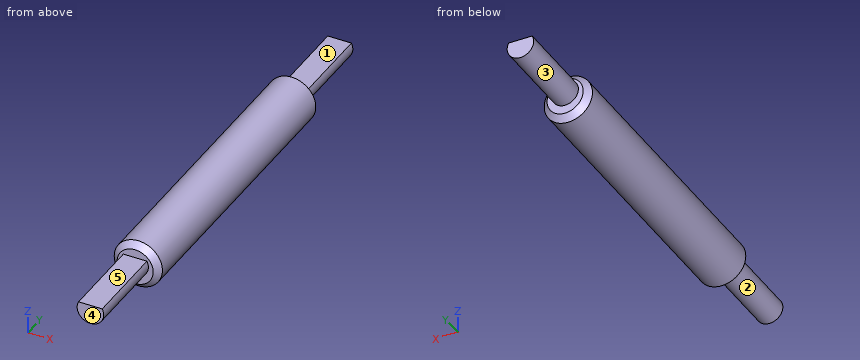
Autodesk Inventor part; units mm, degrees
ref_plane "XZ Plane" through (0, 0, 0) normal (0, 1, 0) x (-1, 0, 0)
ref_plane "XY Plane" through (0, 0, 0) normal (0, 0, 1) x (1, 0, 0)
sketch "Sketch1" plane through (0, 0, 0) normal (0, 1, 0) x (-1, 0, 0)
  circle A0 centre (0, 0) radius 2
  dimension "d0" = 4
extrude "Extrusion1" add sketch "Sketch1" along normal blind 25
sketch "Sketch2" plane through (0, 25, 0) normal (0, 1, 0) x (1, 0, 0)
  line L0 (0, -2) -> (2.3553, -2)
  line L1 (-0.9798, -0.8) -> (0.9798, -0.8)
  arc A0 (0.9798, -0.8) -> (-0.9798, -0.8) centre (0, -0.3) ccw
  circle A1 centre (0, 0) radius 2
  line L2 (3.2263, 0) -> (-2.8711, 0)
  dimension "d4" = 1.2
  dimension "d6" = 1.1
  dimension "d7" = 0.3
extrude "Extrusion2" add sketch "Sketch2" along normal blind 7 contours A0 L2 L1 | A0 L2
sketch "Sketch3" plane through (0, 0, 0) normal (0, -1, 0) x (1, 0, 0)
  line L0 (-0.9798, 0.8) -> (0.9798, 0.8)
  arc A0 (-0.9798, 0.8) -> (0.9798, 0.8) centre (0, 0.3) ccw
  point P0 (0, 0)
  point P1 (0, 0)
  point P2 (0, 0.8)
  dimension "d12" = 1.9596
  dimension "d16" = 1.1
  dimension "d17" = 0.3
extrude "Extrusion3" add sketch "Sketch3" along normal blind 7
chamfer "Chamfer1" distance 0.5 angle 45 1 edges at (2, 25, 0)
chamfer "Chamfer2" distance 0.5 angle 45 1 edges at (2, 0, 0)
equation "\"d4\" = d3"
properties part number "axle-skibidi"
Check sheet for the modelled part. Datum: model origin and axes. Units: mm. Face numbers are marked on the shaded views. A direction names the side the tool comes from. Coordinates: 2 decimals unless noted, no trailing zeros. Loops run counter-clockwise (first coordinate to the right, second up) from the corner with the lowest first, then second, coordinate; pieces in that order, holes last. Notation, with made-up numbers: (-23.5, -27) -> (11.5, -27) arc R21 ccw to (11.5, -5) -> close; hole circle Ø5 at (89, -5.75). An arc over 180 degrees is marked (long way). Write item = value, one per line. Start each with the question number.
1. Tool access check on the marked faces 1, 2, 3, 4 and 5. Record the directions out of +Z, -Z, +X, -X, +Y, -Y that give a thin tool (end or side, any length) a straight path to the whole face; none if there is none.
2. Material ranges on line 1 (Y direction, x = -1.4, z = 0.5); line 2 (Z direction, x = -0.5, y = 18.5); line 3 (Z direction, x = -0.9, y = 1.5), recorded low to high.
3. Section check D-D on y = 22.5. Record the cut outline in (x, z), then the cut area to 3 significant figures.
4. Depth check by flat-ended pin: P1, Ø2, axis at x = -0.5, y = 27, coming from the +Z side. Enter the tip coordinate at first touch or a pass-through.
5. Section check A-A on x = 0. Record the cut outline in (y, z).
6. Section check C-C on y = -2. Record the cut outline in (x, z), then the cut area to 3 significant figures.
7. Section check B-B on z = 0. Record the cut outline in (x, y), then the cut area to 3 significant figures.
Responses:
q1.face_1 = +Z, +X, -X, +Y
q1.face_2 = -Y
q1.face_3 = +Y
q1.face_4 = +Z, -Z, +X, -X, -Y
q1.face_5 = +Z, +X, -X, -Y
q2.line_1 = 0 to 25
q2.line_2 = -1.94 to 1.94
q2.line_3 = -1.79 to 1.79
q3.outline = circle Ø4 at (0, 0)
q3.area = 12.6 mm2
q4.P1 = 0.8
q5.outline = (-7, -0.8) -> (0, -0.8) -> (0, -1.5) -> (0.5, -2) -> (24.5, -2) -> (25, -1.5) -> (25, -0.8) -> (32, -0.8) -> (32, 0.8) -> (25, 0.8) -> (25, 1.5) -> (24.5, 2) -> (0.5, 2) -> (0, 1.5) -> (0, 0.8) -> (-7, 0.8) -> close
q6.outline = (-0.98, 0.8) arc R1.1 ccw (long way) to (0.98, 0.8) -> close
q6.area = 2.96 mm2
q7.outline = (-2, 0.5) -> (-1.5, 0) -> (-1.06, 0) -> (-1.06, -7) -> (1.06, -7) -> (1.06, 0) -> (1.5, 0) -> (2, 0.5) -> (2, 24.5) -> (1.5, 25) -> (1.06, 25) -> (1.06, 32) -> (-1.06, 32) -> (-1.06, 25) -> (-1.5, 25) -> (-2, 24.5) -> close
q7.area = 129 mm2
